For this review, take the finished solid that the model builds, in its own axes (mm). A direction names the side the tool comes from. Coordinates: 2 decimals unless noted, no trailing zeros. Write item = value, one per line.
from build123d import *


with BuildPart() as part:
    # Sketch1 → Revolve-Thin1 (revolve)
    with BuildSketch(Plane.XY, mode=Mode.PRIVATE) as revolve_thin1_sk:
        with BuildLine():
            Line((-76.2, -267.162329894), (-76.2, -292.562329894))
            Line((-76.2, -292.562329894), (-83.82, -292.562329894))
            Line((-83.82, -292.562329894), (-83.82, -305.262329894))
            Line((-83.82, -305.262329894), (-10.081210505, -305.262329894))
            Line((-10.081210505, -305.262329894), (-10.081210505, 469.437670106))
            Line((-10.081210505, 469.437670106), (-35.481210505, 469.437670106))
            ThreePointArc((-35.481210505, 469.437670106), (-66.318439793, 101.716878278), (-76.2, -267.162329894))
        make_face()
        with BuildLine():
            Line((-73.66, -267.160221674), (-73.66, -295.102329894))
            Line((-73.66, -295.102329894), (-81.28, -295.102329894))
            Line((-81.28, -295.102329894), (-81.28, -302.722329894))
            Line((-81.28, -302.722329894), (-12.621210505, -302.722329894))
            Line((-12.621210505, -302.722329894), (-12.621210505, 466.897670106))
            Line((-12.621210505, 466.897670106), (-33.210714263, 466.897670106))
            ThreePointArc((-33.210714263, 466.897670106), (-63.844918494, 100.442329278), (-73.66, -267.160221674))
        make_face(mode=Mode.SUBTRACT)
    revolve(revolve_thin1_sk.sketch.rotate(Axis((0, 0, 0), (0, 1, 0)), 270), axis=Axis((0, 0, 0), (0, 1, 0)))


solid = part.part
Q1. Draft analysis for pull direction X (two halves, no side actions). For faces 4 (the face through (-9.995, 87.511, 1.312)), 5 (the face through (-70.68, -299, -45.06)), 6 (the face through (17, -305.262, 1)), state which applies: +X half, -X half, draft (parallel to the pull), parting line (faces both ways), or undercut.
Solved:
face_4 = undercut
face_5 = parting line
face_6 = draft
Q2. For pin 1 Ø5 at (x, y) = (40, 65.5) entering from +Z; pin 2 Ø3 at (x, y) = (45, -205.5) entering from -Z; pin 3 Ø6 at (y, z) = (-45.5, 62.5) entering from +X, all flat-tipped, find the tip position at first contact; note any pin that passes through.
Solved:
pin_1 = 56.99
pin_2 = -62.33
pin_3 = 41.92
Q3. For line 1 along X through (y, z) = (-296, 0); line 2 along Y through (x, z) = (23, -16); line 3 along X through (y, z) = (-289, 0), list the stretches that pass through material, from the lowest coordinate up.
Solved:
line_1 = -83.82 to -81.28, -12.62 to -10.08, 10.08 to 12.62, 81.28 to 83.82
line_2 = -305.26 to -302.72, 466.9 to 469.44
line_3 = -76.2 to -73.66, -12.62 to -10.08, 10.08 to 12.62, 73.66 to 76.2
Q4. Machinability: for faces 1 (the face through (44.821, -281.327, 58.454)), 2 (the face through (7.4, 469.438, 7.4)), 3 (the face through (46.367, -280.04, 60.47)), which of the approach directions +Z, -Z, +X, -X, +Y, -Y give a long, thin tool a straight path to every point of the face, cutting with its end or side? Answer none if there is none.
Solved:
face_1 = none
face_2 = +Z, -Z, +X, -X, +Y
face_3 = +Y
Q5. Add section A-A (z = 0). State how many separate pieces and enclosed holes the cut face has, and give its area (3 significant figures).
Solved:
separate_pieces = 2
enclosed_holes = 2
area = 8,370 mm²
